Verification items for the finished model (mm, model axes). Round coordinates to 2 decimals unless told otherwise and drop trailing zeros. Loops run counter-clockwise (first coordinate to the right, second up) from the corner with the lowest first, then second, coordinate; pieces in that order, holes last. Notation, with made-up numbers: (31, -15) -> (64, -15) arc R12 cw to (64, 8) -> close; hole circle Ø3 at (20, 81.5). An arc over 180 degrees is marked (long way). Use a Markdown table: item, result. Add a question column.
```python
from build123d import *

# Parameters (mm, degrees)
ESBO_O1_R                = 5
RESSALTO_EXTRUS_O1_DEPTH = 1


with BuildPart() as part:
    # Esboço1 → Ressalto-extrusão1 (new body)
    with BuildSketch(Plane.XY):
        with BuildLine():
            Line((-87.5, 318.171952776), (-120, 318.171952776))
            Line((-120, 318.171952776), (-152.5, 318.171952776))
            Line((-152.5, 318.171952776), (-185, 318.171952776))
            ThreePointArc((-185, 318.171952776), (-199.142135624, 312.3140884), (-205, 298.171952776))
            Line((-205, 298.171952776), (-205, 178.888220282))
            Line((-205, 178.888220282), (-35, 178.888220282))
            Line((-35, 178.888220282), (-35, 298.171952776))
            ThreePointArc((-35, 298.171952776), (-40.857864376, 312.3140884), (-55, 318.171952776))
            Line((-55, 318.171952776), (-87.5, 318.171952776))
        make_face()
        with Locations((-152.5, 198.888220282)):
            Circle(ESBO_O1_R, mode=Mode.SUBTRACT)
        with Locations((-87.5, 198.888220282)):
            Circle(ESBO_O1_R, mode=Mode.SUBTRACT)
        with Locations((-120, 218.888220282)):
            Circle(ESBO_O1_R, mode=Mode.SUBTRACT)
        with Locations((-160, 278.171952776)):
            Circle(ESBO_O1_R, mode=Mode.SUBTRACT)
        with Locations((-80, 278.171952776)):
            Circle(ESBO_O1_R, mode=Mode.SUBTRACT)
    extrude(amount=RESSALTO_EXTRUS_O1_DEPTH)


solid = part.part
```
1) Sectioned sample at A-A on x = -87.5. Enter the section's corners in (y, z), then the cut area to 3 significant figures.
2) Release check for a two-part mould opening along X. For faces 1 (the face through (-120.651, 223.846, 0.493)), 2 (the face through (-198.986, 312.469, 0.493)), 3 (the face through (-121, 250, 0)) record: released by +X, released by -X, zero draft, split by the parting line, or undercut.
3) Thickness scan on line 1 (Y direction, x = -152.5, z = 0.75); line 2 (Y direction, x = -160, z = 0.65); line 3 (X direction, y = 274.5, z = 0.85). Record the ranges inside material, lowest first.
4) Sectioned sample at B-B on z = 0.6. Enter the section's corners in (x, y).
5) Sectioned sample at C-C on x = -117.5. Enter the section's corners in (y, z).
Geometry results:
| question | item | result |
|---|---|---|
| 1 | outline | (178.89, 0) -> (193.89, 0) -> (193.89, 1) -> (178.89, 1) -> close; (203.89, 0) -> (318.17, 0) -> (318.17, 1) -> (203.89, 1) -> close |
| 1 | area | 129 mm^2 |
| 2 | face 1 | undercut |
| 2 | face 2 | released by -X |
| 2 | face 3 | zero draft |
| 3 | line 1 | 178.89 to 193.89, 203.89 to 318.17 |
| 3 | line 2 | 178.89 to 273.17, 283.17 to 318.17 |
| 3 | line 3 | -205 to -163.39, -156.61 to -83.39, -76.61 to -35 |
| 4 | outline | (-205, 178.89) -> (-35, 178.89) -> (-35, 298.17) arc R20 ccw to (-55, 318.17) -> (-185, 318.17) arc R20 ccw to (-205, 298.17) -> close; hole circle Ø10 at (-160, 278.17); hole circle Ø10 at (-152.5, 198.89); hole circle Ø10 at (-120, 218.89); hole circle Ø10 at (-87.5, 198.89); hole circle Ø10 at (-80, 278.17) |
| 5 | outline | (178.89, 0) -> (214.56, 0) -> (214.56, 1) -> (178.89, 1) -> close; (223.22, 0) -> (318.17, 0) -> (318.17, 1) -> (223.22, 1) -> close |
